Geometry: see drawing. Coordinates: mm, zero at the bounding-box minimum. A direction names the side the tool comes from. Round coordinates to 2 decimals unless told otherwise and drop trailing zeros. Loops run counter-clockwise (first coordinate to the right, second up) from the corner with the lowest first, then second, coordinate; pieces in that order, holes last.
(1) Section A-A, the plane y = 1. Return the cut outline in (x, z).
(2) Material intervals for probe 1 along X at (y, z) = (2.25, 24); probe 2 along Z at (x, y) = (4.25, 7.5), sorted ascending.
(3) Section C-C, the plane z = 20. Return the cut outline in (x, y).
(4) Mould query, pull axis Y, two halves, no side actions, for the marked faces 5, 6, 7 and 8. Classes: pulls with the +Y half, pulls with the -Y half, needs draft (parallel to the pull), parting line crosses it, or undercut.
(5) Set-up query: the marked faces 1, 2, 3 and 4. Return all of +Z, -Z, +X, -X, +Y, -Y with unobstructed straight access to the full face (end or side cutting, diameter ignored); none if empty.
(6) Section B-B, the plane x = 4.5. Return the cut outline in (y, z).
(7) First-contact query: pin 1 Ø2 at (x, y) = (2.5, 3.5) entering from -Z; pin 2 Ø1 at (y, z) = (3.5, 18.5) entering from +X; pin 3 Ø4 at (y, z) = (6, 4) entering from -X. Flat tips, straight axial feed; report the tip coordinate or a pass-through.
(8) Section D-D, the plane y = 5.75. Return the cut outline in (x, z), plus the area to 3 significant figures.
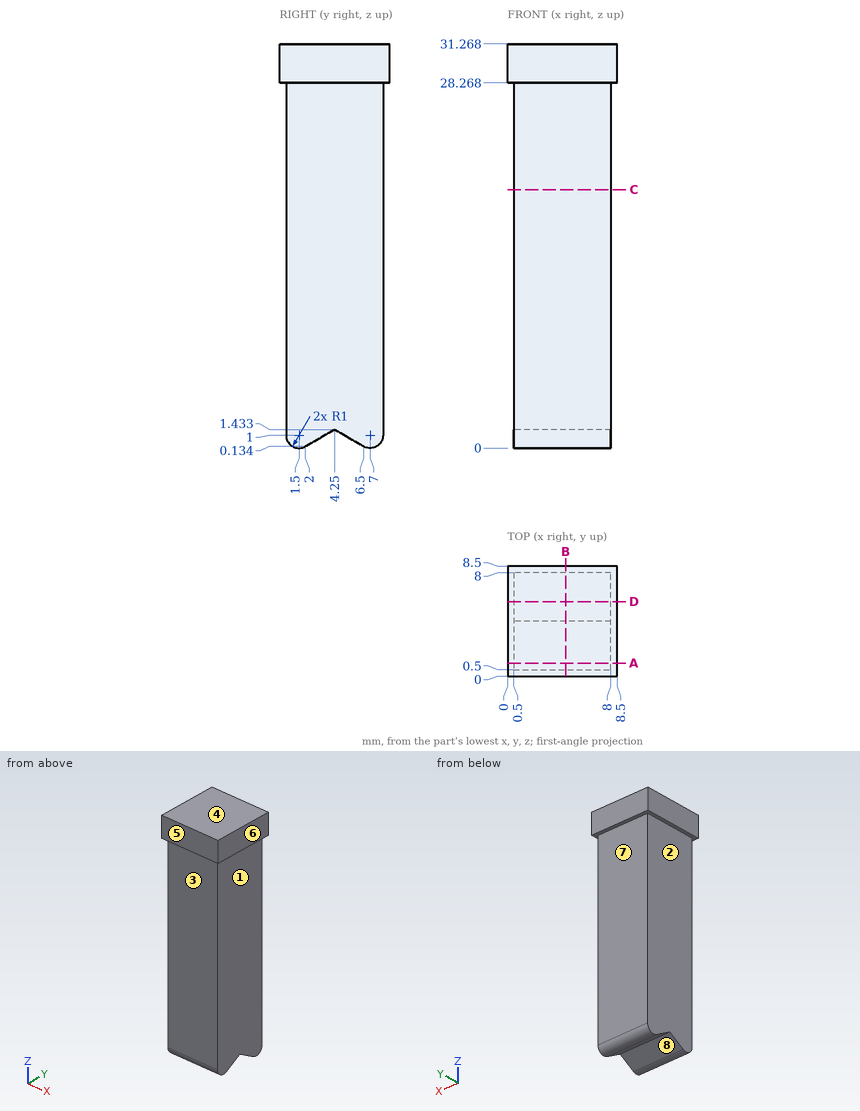
Output values:
1. outline: (0, 28.27) - (0.5, 28.27) - (0.5, 0.13) - (8, 0.13) - (8, 28.27) - (8.5, 28.27) - (8.5, 31.27) - (0, 31.27) - close
2. probe 1: x = 0.5 to 8
2. probe 2: z = 0.13 to 31.27
3. outline: (0.5, 0.5) - (8, 0.5) - (8, 8) - (0.5, 8) - close
4. face 5: pulls with the -Y half
4. face 6: needs draft
4. face 7: pulls with the +Y half
4. face 8: undercut
5. face 1: -Z, +X, +Y, -Y
5. face 2: -Z, -X, +Y, -Y
5. face 3: -Z, +X, -X, -Y
5. face 4: +Z, +X, -X, +Y, -Y
6. outline: (0, 28.27) - (0.5, 28.27) - (0.5, 1) arc R1 ccw to (2, 0.13) - (4.25, 1.43) - (6.5, 0.13) arc R1 ccw to (8, 1) - (8, 28.27) - (8.5, 28.27) - (8.5, 31.27) - (0, 31.27) - close
7. pin 1: stops at z = 0.42
7. pin 2: stops at x = 8
7. pin 3: stops at x = 0.5
8. outline: (0, 28.27) - (0.5, 28.27) - (0.5, 0.57) - (8, 0.57) - (8, 28.27) - (8.5, 28.27) - (8.5, 31.27) - (0, 31.27) - close
8. area: 233 mm2
